Study the drawing (mm; zero at the part's minimum x, y, z) and answer. Round coordinates to 2 decimals unless told otherwise and drop trailing zeros. Order: outer loops, then holes, each group sorted by start corner. A loop starts at its lowest first (then second) coordinate and runs counter-clockwise, first axis right, second up. Notation, with made-up numbers: (-19, 78.5) - (15, 78.5) arc R11 cw to (15, 94.5) - close; hole circle Ø9 at (26.5, 82). An arc over 180 degrees is marked (long way). Put each result on its own line as item: value.
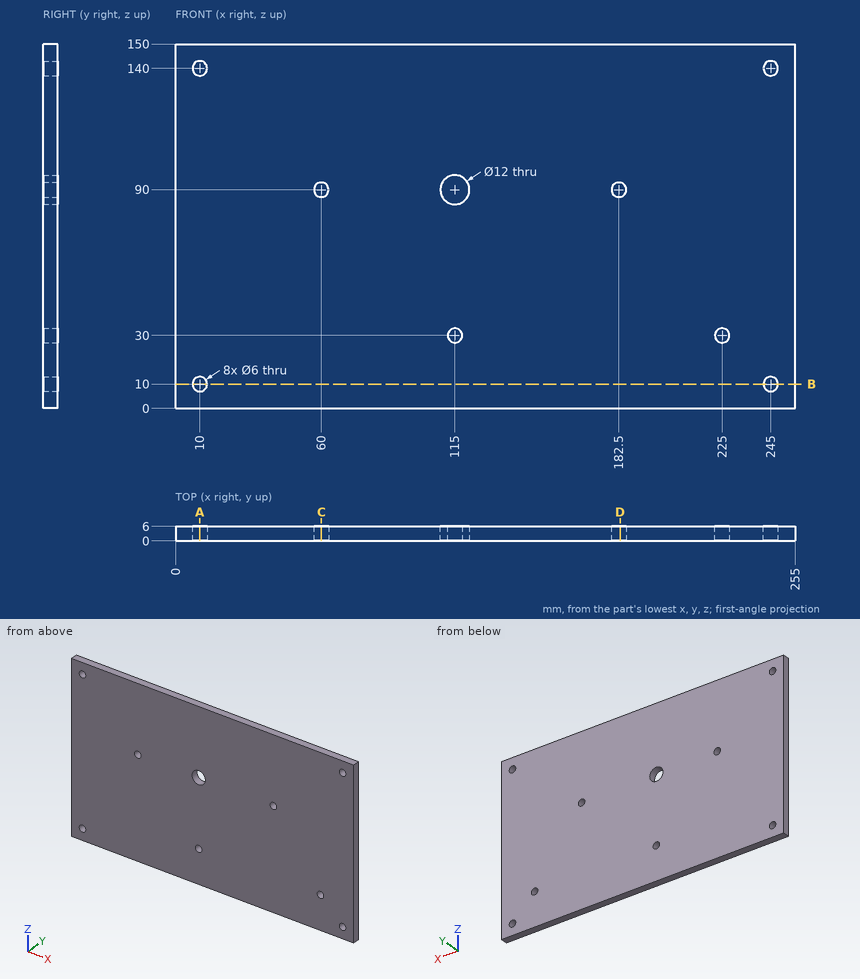
1) A cutting plane is placed at B-B on z = 10. Write down the section's boundary in (x, y), then the cut area to 3 significant figures.
Findings below:
outline: (0, 0) - (7, 0) - (7, 6) - (0, 6) - close; (13, 0) - (242, 0) - (242, 6) - (13, 6) - close; (248, 0) - (255, 0) - (255, 6) - (248, 6) - close
area: 1,460 mm2
2) Given pin 1 Ø5.5 at (x, z) = (10, 140) entering from -Y, flat-ended and moving along its own axis, determine where the tip first touches the part or whether it passes through.
Findings below:
pin 1: passes through
3) A cutting plane is placed at D-D on x = 183. Write down the section's boundary in (y, z), then the cut area to 3 significant figures.
Findings below:
outline: (0, 0) - (6, 0) - (6, 87.04) - (0, 87.04) - close; (0, 92.96) - (6, 92.96) - (6, 150) - (0, 150) - close
area: 865 mm2
4) Straight lines are drawn through the part: L1, parallel to X at y = 2.35, z = 139.5; L2, parallel to Z at x = 245, y = 2.15; L3, parallel to Z at x = 225, y = 2.6. For each, find the intervals that lie inside material, in ascending order. Write a range as from..to.
Findings below:
L1: x = 0..7.04, 12.96..242.04, 247.96..255
L2: z = 0..7, 13..137, 143..150
L3: z = 0..27, 33..150
5) A cutting plane is placed at A-A on x = 10. Write down the section's boundary in (y, z), then the cut area to 3 significant figures.
Findings below:
outline: (0, 0) - (6, 0) - (6, 7) - (0, 7) - close; (0, 13) - (6, 13) - (6, 137) - (0, 137) - close; (0, 143) - (6, 143) - (6, 150) - (0, 150) - close
area: 828 mm2
6) A cutting plane is placed at C-C on x = 60. Write down the section's boundary in (y, z), then the cut area to 3 significant figures.
Findings below:
outline: (0, 0) - (6, 0) - (6, 87) - (0, 87) - close; (0, 93) - (6, 93) - (6, 150) - (0, 150) - close
area: 864 mm2
